```python
from build123d import *

# Parameters (mm, degrees)
SKETCH1_R           = 6.901519969
SKETCH1_R_2         = 6.9
SKETCH1_R_3         = 2.6
BOSS_EXTRUDE1_DEPTH = 5
SKETCH2_R           = 4
SKETCH2_R_2         = 2.6
BOSS_EXTRUDE2_DEPTH = 2


with BuildPart() as part:
    # Sketch1 → Boss-Extrude1 (new body)
    with BuildSketch(Plane.XY):
        with BuildLine():
            Line((-119.047770685, -14.21840763), (-158.491736924, 19.646141241))
            add(Edge.make_bspline(
                [(-158.491736924, 19.646141241), (-160.313597407, 21.050397122), (-161.909962094, 22.656519407)],
                knots=[0, 0, 0, 1, 1, 1], degree=2))
            ThreePointArc((-161.909962094, 22.656519407), (-163.491640093, 26.517106064), (-166.64545249, 29.248278339))
            Line((-166.64545249, 29.248278339), (-169.551288031, 37.112526103))
            ThreePointArc((-169.551288031, 37.112526103), (-180.421756419, 49.833075564), (-181.222431589, 33.119656379))
            Line((-181.222431589, 33.119656379), (-178.794316039, 25.37582765))
            ThreePointArc((-178.794316039, 25.37582765), (-178.212831269, 16.189990788), (-169.857983808, 12.328093938))
            Line((-169.857983808, 12.328093938), (-127.253789064, -21.937441374))
            ThreePointArc((-127.253789064, -21.937441374), (-117.207191003, -24.396487309), (-119.047770685, -14.21840763))
        make_face()
        with Locations((-170.794274728, 21.270925714)):
            Circle(SKETCH1_R, mode=Mode.SUBTRACT)
        with Locations((-177.508495403, 41.317624299)):
            Circle(SKETCH1_R_2, mode=Mode.SUBTRACT)
        with Locations((-121.432089481, -19.905045023)):
            Circle(SKETCH1_R_3, mode=Mode.SUBTRACT)
    extrude(amount=BOSS_EXTRUDE1_DEPTH)

    # Sketch2 → Boss-Extrude2 (add)
    with BuildSketch(Plane.XY.offset(5)):
        with BuildLine():
            Line((-119.047770685, -14.21840763), (-158.491736924, 19.646141241))
            add(Edge.make_bspline(
                [(-158.491736924, 19.646141241), (-160.313597387, 21.050397106), (-161.909962058, 22.656519371)],
                knots=[0, 0, 0, 1, 1, 1], degree=2))
            ThreePointArc((-161.909962058, 22.656519371), (-163.491640057, 26.517106064), (-166.64545249, 29.248278339))
            Line((-166.64545249, 29.248278339), (-169.551288031, 37.112526103))
            ThreePointArc((-169.551288031, 37.112526103), (-180.421756419, 49.833075564), (-181.222431589, 33.119656379))
            Line((-181.222431589, 33.119656379), (-178.794316039, 25.37582765))
            ThreePointArc((-178.794316039, 25.37582765), (-178.212831269, 16.189990788), (-169.857983808, 12.328093938))
            Line((-169.857983808, 12.328093938), (-127.253789064, -21.937441374))
            ThreePointArc((-127.253789064, -21.937441374), (-117.207191003, -24.396487309), (-119.047770685, -14.21840763))
        make_face()
        with Locations((-177.508495403, 41.317624299)):
            Circle(SKETCH2_R, mode=Mode.SUBTRACT)
        with Locations((-170.794274728, 21.270925714)):
            Circle(SKETCH2_R, mode=Mode.SUBTRACT)
        with Locations((-121.432089481, -19.905045023)):
            Circle(SKETCH2_R_2, mode=Mode.SUBTRACT)
    extrude(amount=BOSS_EXTRUDE2_DEPTH)


solid = part.part
```
Design review of the part built by this model. Coordinates are the model's own, in mm. A direction names the side the tool comes from. Coordinates: 2 decimals unless noted, no trailing zeros. Order: outer loops, then holes, each group sorted by start corner. A loop starts at its lowest first (then second) coordinate and runs counter-clockwise, first axis right, second up. Notation, with made-up numbers: (62, -5.5) - (115, -5.5) arc R14 cw to (115, 8.5) - close; hole circle Ø1 at (24.5, 10). An arc over 180 degrees is marked (long way). Answer in a Markdown table with one row per item.
(1) Consider section C-C on x = -139. State the section outline as (y, z) points.
Checked values:
| item | result |
|---|---|
| outline | (-12.49, 0) - (2.91, 0) - (2.91, 7) - (-12.49, 7) - close |
(2) Clearance check with flat-ended pins moving along their axes: pin 1 (18 mm diameter, centred on x = -170.79, y = 21.27, fed in from +Z); pin 2 (4 mm diameter, centred on x = -178, y = 39, fed in from -Z); pin 3 (5 mm diameter, centred on x = -177.51, y = 41.32, fed in from -Z); pin 4 (4 mm diameter, centred on x = -179, z = 2, fed in from -Y). State where each tip first meets the part, or that it passes through.
Checked values:
| item | result |
|---|---|
| pin 1 | z = 7 |
| pin 2 | z = 5 |
| pin 3 | through |
| pin 4 | y = 14.76 |
(3) The part is to be moulded in two halves that separate along X. For faces 1 (the flat face through (-168, 18, 5)), 2 (the cylindrical face through (-124.03, -19.79, 3.45)), 3 (the flat face through (-154, 9, 7)), 4 (the cylindrical face through (-180.136, 49.926, 3.451)), say which applies: released by +X, released by -X, zero draft, split by the parting line, or undercut.
Checked values:
| item | result |
|---|---|
| face 1 | undercut |
| face 2 | undercut |
| face 3 | zero draft |
| face 4 | split by the parting line |
(4) Consider section B-B on z = 2.5. Give the number of separate pieces and of enclosed holes in the cut face, plus the area to 3 significant figures.
Checked values:
| item | result |
|---|---|
| separate pieces | 1 |
| enclosed holes | 3 |
| area | 983 mm^2 |
(5) Consider section D-D on y = -0.5. State the section outline as (x, z) points, plus the area to 3 significant figures.
Checked values:
| item | result |
|---|---|
| outline | (-153.91, 0) - (-135.03, 0) - (-135.03, 7) - (-153.91, 7) - close |
| area | 132 mm^2 |
(6) Wall thickness on line 1 along Y through (x, z) = (-172.5, 3); line 2 along X through (y, z) = (19, 1.75); line 3 along X through (y, z) = (-20, 2.5): over which ranges is each line inside the solid? List them lowest first. Write a range as from..to.
Checked values:
| item | result |
|---|---|
| line 1 | 12.44..14.58, 27.96..36.57, 46.06..48.8 |
| line 2 | -179.49..-177.31, -164.28..-157.74 |
| line 3 | -129.66..-124.03, -118.83..-115.27 |
(7) Consider section A-A on y = -21. State the section outline as (x, z) points, plus the area to 3 significant figures.
Checked values:
| item | result |
|---|---|
| outline | (-128.42, 0) - (-123.79, 0) - (-123.79, 7) - (-128.42, 7) - close; (-119.07, 0) - (-115.36, 0) - (-115.36, 7) - (-119.07, 7) - close |
| area | 58.4 mm^2 |
(8) For faces 5 (the flat face through (-180.025, 29.302, 3.451)), 6 (the cylindrical face through (-181.505, 41.493, 5.986)), 7 (the flat face through (-138.494, 2.477, 3.451)), 8 (the cylindrical face through (-176.27, 17.07, 2.46)), 9 (the flat face through (-168.08, 33.13, 3.45)), list the 3-axis set-ups (+Z, -Z, +X, -X, +Y, -Y) from which the entire face can be reached by the end or side of a thin tool; tool diameter is ignored.
Checked values:
| item | result |
|---|---|
| face 5 | +Z, -Z, -X |
| face 6 | +Z, -Z |
| face 7 | +Z, -Z, +X, +Y |
| face 8 | -Z |
| face 9 | +Z, -Z, +X |
